```python
from build123d import *

# Parameters (mm, degrees)
SKETCH_W          = 292.1
SKETCH_H          = 609.6
PAD_DEPTH         = 19.05
BOX_W             = 3.175
BOX_H             = 609.6
BOX_DEPTH         = 107.95
BOX001_W          = 3.175
BOX001_H          = 609.6
BOX001_DEPTH      = 6.35
CYLINDER_R        = 6.35
CYLINDER_DEPTH    = 6.35
CYLINDER001_R     = 6.35
CYLINDER001_DEPTH = 6.35
CYLINDER002_R     = 6.35
CYLINDER002_DEPTH = 6.35
CYLINDER003_R     = 6.35
CYLINDER003_DEPTH = 6.35
BOX002_W          = 25.4
BOX002_H          = 120.65
BOX002_DEPTH      = 19.05


with BuildPart() as part:
    # Sketch → Pad (new body)
    with BuildSketch(Plane.YZ):
        with Locations((0, 304.8)):
            Rectangle(SKETCH_W, SKETCH_H)
    extrude(amount=PAD_DEPTH)

    # Box → Box (cut)
    with BuildSketch(Plane(origin=(6.35, 133.35, 609.6), x_dir=(0, 1, 0), z_dir=(-1, 0, 0))):
        with Locations((1.5875, 304.8)):
            Rectangle(BOX_W, BOX_H)
    extrude(amount=BOX_DEPTH, mode=Mode.SUBTRACT)

    # Box001 → Box001 (cut)
    with BuildSketch(Plane(origin=(6.35, -136.525, 609.6), x_dir=(0, 1, 0), z_dir=(-1, 0, 0))):
        with Locations((1.5875, 304.8)):
            Rectangle(BOX001_W, BOX001_H)
    extrude(amount=BOX001_DEPTH, mode=Mode.SUBTRACT)

    # Cylinder → Cylinder (cut)
    with BuildSketch(Plane(origin=(6.35, -63.5, 444.5), x_dir=(0, 1, 0), z_dir=(-1, 0, 0))):
        Circle(CYLINDER_R)
    extrude(amount=CYLINDER_DEPTH, mode=Mode.SUBTRACT)

    # Cylinder001 → Cylinder001 (cut)
    with BuildSketch(Plane(origin=(6.35, 38.1, 444.5), x_dir=(0, 1, 0), z_dir=(-1, 0, 0))):
        Circle(CYLINDER001_R)
    extrude(amount=CYLINDER001_DEPTH, mode=Mode.SUBTRACT)

    # Cylinder002 → Cylinder002 (cut)
    with BuildSketch(Plane(origin=(6.35, 38.1, 190.5), x_dir=(0, 1, 0), z_dir=(-1, 0, 0))):
        Circle(CYLINDER002_R)
    extrude(amount=CYLINDER002_DEPTH, mode=Mode.SUBTRACT)

    # Cylinder003 → Cylinder003 (cut)
    with BuildSketch(Plane(origin=(6.35, -63.5, 190.5), x_dir=(0, 1, 0), z_dir=(-1, 0, 0))):
        Circle(CYLINDER003_R)
    extrude(amount=CYLINDER003_DEPTH, mode=Mode.SUBTRACT)

    # Box002 → Box002 (cut)
    with BuildSketch(Plane(origin=(19.05, -57.15, 609.6), x_dir=(0, 1, 0), z_dir=(-1, 0, 0))):
        with Locations((12.7, 60.325)):
            Rectangle(BOX002_W, BOX002_H)
    extrude(amount=BOX002_DEPTH, mode=Mode.SUBTRACT)


solid = part.part
```
Here's how the part is built. I have some questions about the finished solid (model axes, mm). A direction names the side the tool comes from. Coordinates: 2 decimals unless noted, no trailing zeros. Order: outer loops, then holes, each group sorted by start corner. A loop starts at its lowest first (then second) coordinate and runs counter-clockwise, first axis right, second up. Notation, with made-up numbers: (46.25, -4) - (102.25, -4) arc R26 ccw to (102.25, 31) - close; hole circle Ø11 at (-27.5, 76.25). An arc over 180 degrees is marked (long way). One line per question, with ' | ' between items.
(1) Will this pin go through, and if not, where does the flat tip stop? pin 1 (4 mm diameter, centred on y = 40.5, z = 188, fed in from -X).
Report:
pin 1: stops at x = 6.35
(2) If I drill on L1, parallel to Z at x = 2.75, y = 38.1; L2, parallel to Y at x = 2, z = 566.5 (3 decimals); L3, parallel to Y at x = 2, z = 190.5 (3 decimals), over which ranges is the centre line in solid material (lowest first)?
Report:
L1: z = 0 to 184.15, 196.85 to 438.15, 450.85 to 609.6 | L2: y = -146.05 to -136.525, -133.35 to -57.15, -31.75 to 133.35, 136.525 to 146.05 | L3: y = -146.05 to -136.525, -133.35 to -69.85, -57.15 to 31.75, 44.45 to 133.35, 136.525 to 146.05
(3) Suppose I cut it at A-A on z = 500. List the corners of the cut face in (x, y) for me (3 decimals).
Report:
outline: (0, -146.05) - (19.05, -146.05) - (19.05, -57.15) - (0, -57.15) - (0, -133.35) - (6.35, -133.35) - (6.35, -136.525) - (0, -136.525) - close; (0, -31.75) - (19.05, -31.75) - (19.05, 146.05) - (0, 146.05) - (0, 136.525) - (6.35, 136.525) - (6.35, 133.35) - (0, 133.35) - close
(4) For faces 5 (the flat face through (6.35, 38, 190)), 6 (the flat face through (10, -31.75, 550)), 7 (the flat face through (0, -2, 309)), which set-ups out of +Z, -Z, +X, -X, +Y, -Y let a thin tool reach every point of the face, with its end or its side?
Report:
face 5: -X | face 6: +Z, +X, -X | face 7: +Z, -Z, -X, +Y, -Y
(5) Suppose I cut it at D-D on y = -49.5. List the corners of the cut face in (x, z) for me, and give its area (3 significant figures).
Report:
outline: (0, 0) - (19.05, 0) - (19.05, 488.95) - (0, 488.95) - close | area: 9,310 mm2
(6) If we mould it in two halves opening along Z, with no side actions, what happens to faces 1 (the cylindrical face through (3.22, 36.72, 450.7)), 2 (the flat face through (10, -45, 488.95)), 3 (the flat face through (6.35, -64, 190)), 4 (the flat face through (19.05, -2, 309))? For each: pulls with the +Z half, pulls with the -Z half, needs draft (parallel to the pull), parting line crosses it, or undercut.
Report:
face 1: undercut | face 2: pulls with the +Z half | face 3: undercut | face 4: needs draft
(7) Suppose I cut it at B-B on x = 10.75. List the corners of the cut face in (y, z) for me, and give its area (3 significant figures).
Report:
outline: (-146.05, 0) - (146.05, 0) - (146.05, 609.6) - (-31.75, 609.6) - (-31.75, 488.95) - (-57.15, 488.95) - (-57.15, 609.6) - (-146.05, 609.6) - close | area: 175,000 mm2
(8) Suppose I cut it at C-C on z = 190.5. List the corners of the cut face in (x, y) for me (3 decimals).
Report:
outline: (0, -146.05) - (19.05, -146.05) - (19.05, 146.05) - (0, 146.05) - (0, 136.525) - (6.35, 136.525) - (6.35, 133.35) - (0, 133.35) - (0, 44.45) - (6.35, 44.45) - (6.35, 31.75) - (0, 31.75) - (0, -57.15) - (6.35, -57.15) - (6.35, -69.85) - (0, -69.85) - (0, -133.35) - (6.35, -133.35) - (6.35, -136.525) - (0, -136.525) - close
